Can you work these out from the drawing? Everything is in mm from the part's minimum corner. Round coordinates to 2 decimals unless told otherwise and drop trailing zeros. Write each loop counter-clockwise with the first axis right and the second up, starting at its lowest first coordinate (ties: lowest second). Pieces come first, ordered by that corner, then holes. Notation, with made-up numbers: (55.5, -3.75) -> (86.5, -3.75) arc R17 cw to (86.5, 7.25) -> close; hole circle Ø4 at (-26, 18). An arc over 180 degrees is marked (long way). Answer as CSV lines item,"result". Start each with the question number.
Q1. Will these pins go through, and if not, where does the flat tip stop? pin 1 Ø1 at (x, y) = (22, 47.5) entering from -Z; pin 2 Ø5 at (x, y) = (30, 10) entering from +Z; pin 3 Ø1.5 at (x, z) = (33.5, 2) entering from +Y; pin 4 Ø7 at (x, y) = (10, 50) entering from +Z.
Q2. If I drill on line 1 (Y direction, x = 10, z = 0.45); line 2 (Y direction, x = 30, z = 1.25); line 3 (X direction, y = 52.5, z = 2), over which ranges is the centre line in solid material (lowest first)? Write a range as [from, to].
Q3. Imagine slicing it at A-A on y = 10. Please give me the cut outline in (x, z), and give its area (3 significant figures).
Q4. Imagine slicing it at B-B on x = 50. Please give me the cut outline in (y, z).
Q5. If we mould it in two halves opening along X, with no side actions, what happens to the marked faces 1, 2 and 3? For each: pulls with the +X half, pulls with the -X half, needs draft (parallel to the pull), parting line crosses it, or undercut.
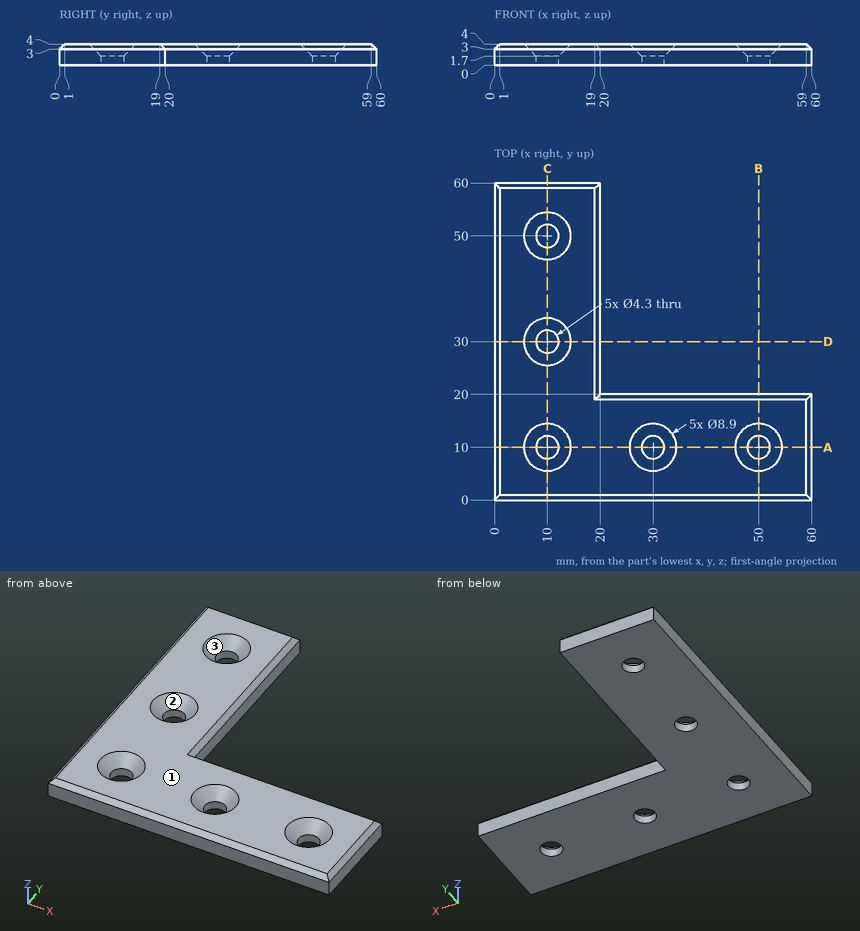
Checks:
1,pin 1,"through"
1,pin 2,"z = 2.05"
1,pin 3,"y = 20"
1,pin 4,"z = 3.05"
2,line 1,"[0, 7.85], [12.15, 27.85], [32.15, 47.85], [52.15, 60]"
2,line 2,"[0, 7.85], [12.15, 20]"
2,line 3,"[0, 20]"
3,outline,"(0, 0) -> (7.85, 0) -> (7.85, 1.7) -> (5.55, 4) -> (1, 4) -> (0, 3) -> close; (12.15, 0) -> (27.85, 0) -> (27.85, 1.7) -> (25.55, 4) -> (14.45, 4) -> (12.15, 1.7) -> close; (32.15, 0) -> (47.85, 0) -> (47.85, 1.7) -> (45.55, 4) -> (34.45, 4) -> (32.15, 1.7) -> close; (52.15, 0) -> (60, 0) -> (60, 3) -> (59, 4) -> (54.45, 4) -> (52.15, 1.7) -> close"
3,area,"172 mm^2"
4,outline,"(0, 0) -> (7.85, 0) -> (7.85, 1.7) -> (5.55, 4) -> (1, 4) -> (0, 3) -> close; (12.15, 0) -> (20, 0) -> (20, 3) -> (19, 4) -> (14.45, 4) -> (12.15, 1.7) -> close"
5,face 1,"needs draft"
5,face 2,"undercut"
5,face 3,"undercut"
